Source: three-view drawing plus pictorial views. Frame: mm from the lowest corner of the part. A direction names the side the tool comes from. Give positions to 0.01 mm unless a question says otherwise; leave off trailing zeros. Loops run counter-clockwise (first coordinate to the right, second up) from the corner with the lowest first, then second, coordinate; pieces in that order, holes last. Notation, with made-up numbers: (-2.75, -31) - (17.25, -31) arc R23 ccw to (17.25, -19) - close; hole circle Ø4 at (-7, 21). An arc over 180 degrees is marked (long way). One line per item, written item: value.
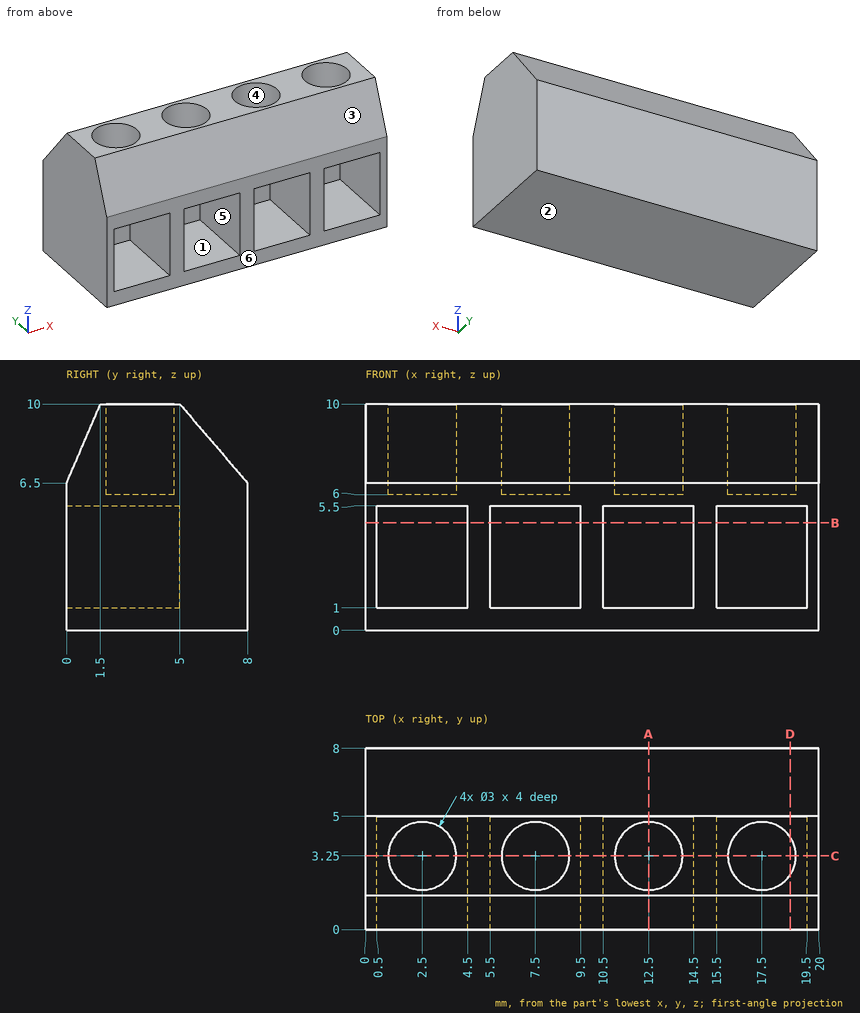
Item 1: Section A-A, the plane x = 12.5. Output: boundary loops of the cut face in (y, z), and give its area (3 significant figures).
Verdict:
outline: (0, 0) - (8, 0) - (8, 6.5) - (5, 10) - (4.75, 10) - (4.75, 6) - (1.75, 6) - (1.75, 10) - (1.5, 10) - (0, 6.5) - (0, 5.5) - (5, 5.5) - (5, 1) - (0, 1) - close
area: 37.6 mm^2
Item 2: Draft query along Z for the marked faces 1, 2 and 3. Return one class per face: pulls with the +Z half, pulls with the -Z half, needs draft (parallel to the pull), parting line crosses it, or undercut.
Verdict:
face 1: undercut
face 2: pulls with the -Z half
face 3: pulls with the +Z half
Item 3: Pin query (flat end, axial travel): P1, Ø0.9, axis at x = 8, y = 2.5, coming from the +Z side. Return the tip coordinate at first contact, or that it passes through.
Verdict:
P1: stops at z = 6
Item 4: Section C-C, the plane y = 3.25. Count the separate pieces of the cut face and the enclosed holes in it, and give its area (3 significant figures).
Verdict:
separate pieces: 1
enclosed holes: 4
area: 80.0 mm^2
Item 5: Section B-B, the plane z = 4.75. Output: boundary loops of the cut face in (x, y).
Verdict:
outline: (0, 0) - (0.5, 0) - (0.5, 5) - (4.5, 5) - (4.5, 0) - (5.5, 0) - (5.5, 5) - (9.5, 5) - (9.5, 0) - (10.5, 0) - (10.5, 5) - (14.5, 5) - (14.5, 0) - (15.5, 0) - (15.5, 5) - (19.5, 5) - (19.5, 0) - (20, 0) - (20, 8) - (0, 8) - close
Item 6: Material intervals for L1, parallel to X at y = 4, z = 4.5; L2, parallel to Z at x = 18.25, y = 2; L3, parallel to Z at x = 10.75, y = 4.5, sorted ascending.
Verdict:
L1: x = 0 to 0.5, 4.5 to 5.5, 9.5 to 10.5, 14.5 to 15.5, 19.5 to 20
L2: z = 0 to 1, 5.5 to 6
L3: z = 0 to 1, 5.5 to 10
Item 7: Access query for the marked faces 4, 5 and 6. Directions: +Z, -Z, +X, -X, +Y, -Y. A direction counts if a zero-diameter tool reaches every point of the face in a straight line with its end or side. Return the directions, or none.
Verdict:
face 4: +Z
face 5: -Y
face 6: +Z, -Z, +X, -X, -Y
Item 8: Section D-D, the plane x = 18.75. Output: boundary loops of the cut face in (y, z), and give its area (3 significant figures).
Verdict:
outline: (0, 0) - (8, 0) - (8, 6.5) - (5, 10) - (4.08, 10) - (4.08, 6) - (2.42, 6) - (2.42, 10) - (1.5, 10) - (0, 6.5) - (0, 5.5) - (5, 5.5) - (5, 1) - (0, 1) - close
area: 43.0 mm^2
